Model file for the job. Use its own axes, mm. A direction names the side the tool comes from. Give positions to 0.01 mm unless a question says otherwise; leave off trailing zeros. Write each loop counter-clockwise with the first axis right and the second up, starting at its lowest first coordinate (ties: lowest second). Pieces come first, ordered by that corner, then holes. Notation, with made-up numbers: (64.25, 75) - (115.25, 75) arc R27 ccw to (115.25, 99) - close; hole circle Ø6 at (-3, 51). An arc over 180 degrees is marked (long way). One line per item, written item: value. Start each with the question number.
(1) Cut at C-C, the plane x = 10.25. List the corners of the cut face in (y, z).
(2) Drop a flat-ended pin along its axis: P1, Ø3, axis at x = 8, y = 4, coming from the -Z side. Give the stop position or say it passes through.
(3) 3-axis set-ups, long thin cutter, end or side, ignore diameter. For faces 4 (the face through (6, -5, 15)), 5 (the face through (12, 13, 0)): which of +Z, -Z, +X, -X, +Y, -Y reach the whole face in a straight line?
(4) Cut at A-A, the plane z = 15. List the corners of the cut face in (x, y), and give its area (3 significant figures).
(5) Mould opens along X. For faces 1 (the face through (1.25, 13, 15)), 2 (the face through (-5.537, 36.748, 19.72)), 3 (the face through (6, 13, 40)) say: pulls with the +X half, pulls with the -X half, needs draft (parallel to the pull), parting line crosses it, or undercut.
(6) Probe L1, parallel to X at y = 7.5, z = 16; L2, parallel to Y at x = 10.75, z = 23.5; L3, parallel to Z at x = 4, y = 19.5. List the from-to ranges inside material, lowest first.
(7) Cut at B-B, the plane y = 23.5. List the corners of the cut face in (x, z).
Autodesk Inventor part; units mm, degrees
ref_plane "YZ Plane" through (0, 0, 0) normal (1, 0, 0) x (0, 1, 0)
ref_plane "XZ Plane" through (0, 0, 0) normal (0, 1, 0) x (-1, 0, 0)
ref_plane "XY Plane" through (0, 0, 0) normal (0, 0, 1) x (1, 0, 0)
sketch "Sketch1" plane through (0, 0, 0) normal (0, 0, 1) x (1, 0, 0)
  line L0 (11.25, -5) -> (1.25, -5)
  line L1 (1.25, -5) -> (1.25, 30)
  line L2 (1.25, 30) -> (11.25, 30)
  line L3 (11.25, 30) -> (11.25, -5)
  arc A0 (16.25, -12.5) -> (18.75, -10) centre (16.25, -10) ccw
  line L4 (18.75, -10) -> (18.75, 35)
  arc A1 (18.75, 35) -> (16.25, 37.5) centre (16.25, 35) ccw
  line L5 (16.25, 37.5) -> (-3.75, 37.5)
  arc A2 (-3.75, 37.5) -> (-6.25, 35) centre (-3.75, 35) ccw
  line L6 (-6.25, 35) -> (-6.25, -10)
  arc A3 (-6.25, -10) -> (-3.75, -12.5) centre (-3.75, -10) ccw
  line L7 (-3.75, -12.5) -> (16.25, -12.5)
  line L8 (-6.25, -10) -> (-6.25, 35)
  arc A4 (-3.75, 37.5) -> (-6.25, 35) centre (-3.75, 35) ccw
  line L9 (-3.75, 37.5) -> (16.25, 37.5)
  arc A5 (18.75, 35) -> (16.25, 37.5) centre (16.25, 35) ccw
  line L10 (18.75, 35) -> (18.75, -10)
  arc A6 (16.25, -12.5) -> (18.75, -10) centre (16.25, -10) ccw
  line L11 (16.25, -12.5) -> (-3.75, -12.5)
  arc A7 (-6.25, -10) -> (-3.75, -12.5) centre (-3.75, -10) ccw
  point P0 (0, 0)
  dimension "d0" = 0
extrude "Extrusion1" add sketch "Sketch1" along normal blind 40 contours L0 L1 L2 L3 | L7 A3 L6 A2 L5 A1 L4 A0
sketch "Sketch2" plane through (0, 0, 0) normal (0, 0, -1) x (-1, 0, 0)
  line L0 (-16.25, -10) -> (-16.25, 35)
  line L1 (3.75, -10) -> (-16.25, -10)
  line L2 (3.75, 35) -> (3.75, -10)
  line L3 (-16.25, 35) -> (3.75, 35)
  line L4 (-11.25, -5) -> (-11.25, 30)
  line L5 (-11.25, 30) -> (-1.25, 30)
  line L6 (-1.25, 30) -> (-1.25, -5)
  line L7 (-1.25, -5) -> (-11.25, -5)
  line L8 (-2.75, 28.5) -> (-9.75, 28.5)
  line L9 (-9.75, 28.5) -> (-9.75, -3.5)
  line L10 (-9.75, -3.5) -> (-2.75, -3.5)
  line L11 (-2.75, -3.5) -> (-2.75, 28.5)
  line L12 (-1.25, -5) -> (-11.25, -5)
  line L13 (-11.25, -5) -> (-11.25, 30)
  line L14 (-11.25, 30) -> (-1.25, 30)
  line L15 (-1.25, 30) -> (-1.25, -5)
  point P0 (0, 0)
extrude "Extrusion2" cut sketch "Sketch2" against normal blind 30 contours L4 L5 L6 L7 | L11 L10 L9 L8
properties part number "USB_Cap"
Answers follow:
1. outline: (-12.5, 0) - (-5, 0) - (-5, 30) - (30, 30) - (30, 0) - (37.5, 0) - (37.5, 40) - (-12.5, 40) - close
2. P1: stops at z = 30
3. face 4: -Z
3. face 5: -Z, +X, -X, +Y, -Y
4. outline: (-6.25, -10) arc R2.5 ccw to (-3.75, -12.5) - (16.25, -12.5) arc R2.5 ccw to (18.75, -10) - (18.75, 35) arc R2.5 ccw to (16.25, 37.5) - (-3.75, 37.5) arc R2.5 ccw to (-6.25, 35) - close; hole (1.25, -5) - (11.25, -5) - (11.25, 30) - (1.25, 30) - close
4. area: 895 mm²
5. face 1: undercut
5. face 2: pulls with the -X half
5. face 3: needs draft
6. L1: x = -6.25 to 1.25, 11.25 to 18.75
6. L2: y = -12.5 to -5, 30 to 37.5
6. L3: z = 30 to 40
7. outline: (-6.25, 0) - (1.25, 0) - (1.25, 30) - (11.25, 30) - (11.25, 0) - (18.75, 0) - (18.75, 40) - (-6.25, 40) - close
